from build123d import *

# Parameters (mm, degrees)
F1_DEPTH      = 25
F2_R          = 2
F3_DEPTH      = 25
F3_DEPTH_BACK = 25
F4_START      = 5
F4_DEPTH      = 20
F6_START      = 20
F5_R          = 2
F6_DEPTH      = 20
F7_DEPTH      = 40
F8_R          = 5


with BuildPart() as f1:
    # F0 (on Front) → F1 (new body)
    with BuildSketch(Plane.XZ):
        Polygon((0, 15), (0, 0), (40, 0), (40, 5), (0, 28), (-40, 28), (-40, 15), align=None)
    extrude(amount=-F1_DEPTH)

    # F2 (on Top) → F3 (cut, two sides)
    with BuildSketch(Plane.XY) as f3_sk:
        with Locations((30, 12.5)):
            Circle(F2_R)
        with Locations((15, 12.5)):
            Circle(F2_R)
    extrude(amount=F3_DEPTH, mode=Mode.SUBTRACT)
    extrude(f3_sk.sketch, amount=-F3_DEPTH_BACK, mode=Mode.SUBTRACT)

    # F2 (on Top) → F4 (cut)
    with BuildSketch(Plane.XY.offset(F4_START)):
        Polygon((11.5, 14.5207259422), (11.5, 10.4792740578), (15, 8.4585481157), (18.5, 10.4792740578), (18.5, 14.5207259422), (15, 16.5414518843), align=None)
        with Locations((15, 12.5)):
            Circle(F2_R, mode=Mode.SUBTRACT)
        Polygon((26.5, 14.5207259422), (26.5, 10.4792740578), (30, 8.4585481157), (33.5, 10.4792740578), (33.5, 14.5207259422), (30, 16.5414518843), align=None)
        with Locations((30, 12.5)):
            Circle(F2_R, mode=Mode.SUBTRACT)
    extrude(amount=F4_DEPTH, mode=Mode.SUBTRACT)

    # F5 (on Top) → F6 (cut)
    with BuildSketch(Plane.XY.offset(F6_START)):
        Polygon((-22.9792740578, 21), (-27.0207259422, 21), (-29.0414518843, 17.5), (-27.0207259422, 14), (-22.9792740578, 14), (-20.9585481157, 17.5), align=None)
        with Locations((-25, 17.5)):
            Circle(F5_R, mode=Mode.SUBTRACT)
        Polygon((-22.9792740578, 11), (-27.0207259422, 11), (-29.0414518843, 7.5), (-27.0207259422, 4), (-22.9792740578, 4), (-20.9585481157, 7.5), align=None)
        with Locations((-25, 7.5)):
            Circle(F5_R, mode=Mode.SUBTRACT)
    extrude(amount=F6_DEPTH, mode=Mode.SUBTRACT)

    # F5 (on Top) → F7 (cut)
    with BuildSketch(Plane.XY):
        with Locations((-25, 7.5)):
            Circle(F5_R)
        with Locations((-25, 17.5)):
            Circle(F5_R)
    extrude(amount=F7_DEPTH, mode=Mode.SUBTRACT)

    # F8
    f8_edges = [f1.edges().sort_by_distance(p)[0] for p in [
        (0, 12.5, 15),
    ]]
    fillet(f8_edges, radius=F8_R)


solid = f1.part
Read the model definition and answer for the solid it produces. Units are mm, in the model's axes. A direction names the side the tool comes from. Coordinates: 2 decimals unless noted, no trailing zeros. Loops run counter-clockwise (first coordinate to the right, second up) from the corner with the lowest first, then second, coordinate; pieces in that order, holes last.
Q1. Each of these flat-tipped pins is pushed along its axis until it touches: pin 1 Ø5 at (x, y) = (23.5, 7) entering from +Z (3 decimals); pin 2 Ø1.1 at (y, z) = (13, 6.5) entering from -X; pin 3 Ø4.5 at (y, z) = (13.5, 14) entering from +X. Where does it stop, or does it pass through?
Q2. The part is cut by section D-D on x = 25.5. Write down the section's boundary in (y, z).
Q3. Which of the six approach directions +Z, -Z, +X, -X, +Y, -Y give full straight-line access (tool end or side, diameter ignored) to faces 1 (the face through (-25.26, 19.483, 17.465)), 2 (the face through (-25, 21, 24)), 3 (the face through (-23, 12, 15))?
Q4. The part is cut by section A-A on x = -25. Write down the section's boundary in (y, z).
Q5. The part is cut by section C-C on y = 20.25. Write down the section's boundary in (x, z).
Q6. The mould has two halves that part along X. Classify faces 4 (the face through (14.74, 14.483, 2.465)), 5 (the face through (-1, 25, 14)): +X half, -X half, draft (parallel to the pull), parting line (faces both ways), or undercut.
Q7. Consider probe 1 along Y at (x, z) = (-25, 17.9); probe 2 along X at (y, z) = (14.25, 3.75); probe 3 along Y at (x, z) = (-26.5, 19.75). Determine where each line is inside the solid, lowest interval first.
Q8. The part is cut by section B-B on z = 13.5. Write down the section's boundary in (x, y).
Results below:
1. pin 1: stops at z = 15.925
1. pin 2: stops at x = 0
1. pin 3: stops at x = 27.3
2. outline: (0, 0) - (25, 0) - (25, 13.34) - (0, 13.34) - close
3. face 1: +Z, -Z
3. face 2: +Z
3. face 3: -Z, -X, +Y, -Y
4. outline: (0, 15) - (5.5, 15) - (5.5, 20) - (4, 20) - (4, 28) - (0, 28) - close; (9.5, 15) - (15.5, 15) - (15.5, 20) - (14, 20) - (14, 28) - (11, 28) - (11, 20) - (9.5, 20) - close; (19.5, 15) - (25, 15) - (25, 28) - (21, 28) - (21, 20) - (19.5, 20) - close
5. outline: (-40, 15) - (-5, 15) arc R5 cw to (0, 10) - (0, 0) - (40, 0) - (40, 5) - (0, 28) - (-22.55, 28) - (-22.55, 20) - (-27.45, 20) - (-27.45, 28) - (-40, 28) - close
6. face 4: undercut
6. face 5: draft
7. probe 1: y = 0 to 5.5, 9.5 to 15.5, 19.5 to 25
7. probe 2: x = 0 to 14.03, 15.97 to 29.03, 30.97 to 40
7. probe 3: y = 0 to 6.18, 8.82 to 16.18, 18.82 to 25
8. outline: (-1.43, 0) - (25.22, 0) - (25.22, 25) - (-1.43, 25) - close; hole (11.5, 10.48) - (15, 8.46) - (18.5, 10.48) - (18.5, 14.52) - (15, 16.54) - (11.5, 14.52) - close
